Input: part model. Units: mm. Frame: model coordinates. Coordinates: 2 decimals unless noted, no trailing zeros. Order: outer loops, then holes, each group sorted by start corner. A loop starts at its lowest first (then second) coordinate and runs counter-clockwise, first axis right, second up. Notation, with made-up numbers: (-10, 28) -> (45, 28) arc R26 ccw to (45, 57) -> close; hole circle Ø5 at (52.25, 11). An arc over 180 degrees is marked (long way). Use one line per item in the form item = value. Start each with the question number.
1) Pin query (flat end, axial travel): pin 1 (3 mm diameter, centred on x = 4.5, y = -201, fed in from +Z); pin 2 (1.5 mm diameter, centred on x = 5, z = 2, fed in from -Y); pin 3 (1 mm diameter, centred on x = 5, z = 49, fed in from +Y). Return the tip coordinate at first contact, or that it passes through.
2) Section query A-A on x = 5.25. Output: boundary loops of the cut face in (y, z), then the cut area to 3 significant figures.
3) Section query B-B on y = -34. Output: boundary loops of the cut face in (x, z).
4) Section query C-C on z = 37. Output: boundary loops of the cut face in (x, y).
5) Ray query, line 1 along Z through (x, y) = (2.75, -2); line 2 along Z through (x, y) = (3.75, -242); line 3 along Y through (x, z) = (5.75, -4). Return the intervals inside material, ascending.
Autodesk Inventor part; units mm, degrees
ref_plane "YZ Plane" through (0, 0, 0) normal (1, 0, 0) x (0, 1, 0)
ref_plane "XZ Plane" through (0, 0, 0) normal (0, 1, 0) x (-1, 0, 0)
ref_plane "XY Plane" through (0, 0, 0) normal (0, 0, 1) x (1, 0, 0)
sketch "Sketch1" plane through (0, 0, 0) normal (1, 0, 0) x (0, 1, 0)
  circle A0 centre (0, 0) radius 3.175
  line L0 (0, 0) -> (12.7, 0)
  line L1 (0, 0) -> (12.7, 0) construction
  line L2 (12.7, 0) -> (12.7, -12.7)
  line L3 (12.7, -12.7) -> (-405.9936, -12.7)
  line L4 (-405.9936, -12.7) -> (-405.9936, 12.7)
  line L5 (-405.9936, 12.7) -> (12.7, 12.7)
  line L6 (12.7, 12.7) -> (12.7, -12.7)
  line L7 (-405.9936, 12.7) -> (-498.3106, 105.017)
  line L8 (-405.9936, 12.7) -> (-275.4376, 12.7) construction
  line L9 (-498.3106, 105.017) -> (-516.2711, 87.0565)
  line L10 (-516.2711, 87.0565) -> (-408.5081, -20.7066)
  line L11 (-405.9936, -12.7) -> (-431.3936, -12.7)
  line L12 (-405.9936, -12.7) -> (-380.5936, -12.7) construction
  line L13 (-516.2711, 87.0565) -> (-416.5146, -12.7)
  line L14 (-416.5146, -12.7) -> (12.7, -12.7)
  dimension "d0" = 6.35
  dimension "d1" = 12.7
  dimension "d2" = 0
  dimension "d3" = 12.7
  dimension "d4" = 90
  dimension "d5" = 418.6936
  dimension "d6" = 25.4
  dimension "d7" = 130.556
  dimension "d8" = 135
  dimension "d9" = 25.4
  dimension "d10" = 90
  dimension "d11" = 152.4
  dimension "d12" = 90
  dimension "d13" = 25.4
  dimension "d14" = 180
extrude "Extrusion1" add sketch "Sketch1" along normal blind 25.4
sketch "Sketch2" plane through (25.4, 0, 0) normal (1, 0, 0) x (0, 0, -1)
  line L0 (-105.017, -498.3106) -> (-87.0565, -516.2711)
  line L1 (-87.0565, -516.2711) -> (12.7, -416.5146)
  line L2 (-12.7, 12.7) -> (-12.7, -405.9936)
  line L3 (-96.0368, -507.2909) -> (-78.0763, -507.2909)
  line L4 (-105.017, -498.3106) -> (-100.5269, -502.8008)
  line L5 (-100.5269, -502.8008) -> (-73.5861, -502.8008)
  arc A0 (-100.5269, -502.8008) -> (-73.5861, -502.8008) centre (-87.0565, -489.3304) ccw
  dimension "d17" = 6.35
  dimension "d18" = 19.05
extrude "Extrusion2" cut sketch "Sketch2" against normal blind 25.4 contours A0 L3 L0 | L3 A0 L1 L0 | L1 L3 A0
sketch "Sketch3" plane through (0, 12.7, 12.7) normal (0, 1, 0) x (1, 0, 0)
  line L0 (0, 25.4) -> (0, 0)
  line L1 (0, 0) -> (25.4, 0)
  line L2 (25.4, 25.4) -> (25.4, 0)
  line L3 (0, 25.4) -> (25.4, 25.4)
  point P0 (0, 12.7)
extrude "Extrusion3" add sketch "Sketch3" along normal blind 127
sketch "Sketch4" plane through (25.4, 0, 0) normal (1, 0, 0) x (0, 0, -1)
  arc A0 (-100.5269, -502.8008) -> (-73.5861, -502.8008) centre (-87.0565, -489.3304) ccw
  line L0 (-73.5861, -502.8008) -> (12.7, -416.5146)
  line L1 (12.7, -416.5146) -> (12.7, 139.7)
  line L2 (-12.7, 139.7) -> (12.7, 139.7)
  line L3 (-12.7, -405.9936) -> (-12.7, 139.7)
  line L4 (-12.7, -405.9936) -> (-105.017, -498.3106)
  line L5 (-105.017, -498.3106) -> (-100.5269, -502.8008)
  circle A1 centre (0, 0) radius 3.175
extrude "Extrusion4" cut sketch "Sketch4" against normal blind 19.05
sketch "Sketch5" plane through (6.35, 0, 0) normal (1, 0, 0) x (0, 0, -1)
  line L0 (-12.7, 139.7) -> (12.7, 139.7)
  line L1 (12.7, 139.7) -> (12.7, 12.7)
  line L2 (12.7, 12.7) -> (-12.7, 12.7)
  line L3 (-12.7, 12.7) -> (-12.7, 139.7)
  dimension "d25" = 25.4
  dimension "d26" = 127
extrude "Extrusion5" cut sketch "Sketch5" against normal blind 127
sketch "Sketch8" plane through (6.35, 12.7, 12.7) normal (0, 1, 0) x (1, 0, 0)
  line L0 (-6.35, 0) -> (-6.35, 25.4)
  line L1 (0, 0) -> (-6.35, 0)
  line L2 (0, 25.4) -> (0, 0)
  line L3 (-6.35, 25.4) -> (0, 25.4)
  point P0 (-6.35, 12.7)
extrude "Extrusion8" add sketch "Sketch8" along normal blind 101.6
sketch "Sketch9" plane through (6.35, 0, 0) normal (1, 0, 0) x (0, 0, -1)
  circle A0 centre (0, 0) radius 3.175
  circle A1 centre (0, 0) radius 6.35
  dimension "d45" = 12.7
extrude "Extrusion9" cut sketch "Sketch9" against normal blind 25.4
sketch "Sketch10" plane through (6.35, 0, 0) normal (1, 0, 0) x (0, 0, -1)
  circle A0 centre (0, 0) radius 6.35
  line L0 (-5.5563, -5.5563) -> (5.5563, -5.5563)
  line L1 (5.5563, -5.5563) -> (5.5563, 5.5563)
  line L2 (5.5563, 5.5563) -> (-5.5563, 5.5563)
  line L3 (-5.5563, 5.5563) -> (-5.5563, -5.5563)
  line L4 (-5.5563, -5.5563) -> (5.5563, 5.5563) construction
  line L5 (5.5563, -5.5563) -> (-5.5563, 5.5563) construction
  line L6 (5.5563, -3.0742) -> (0.1158, -6.3489)
  line L7 (0.1158, -6.3489) -> (-5.4404, -3.2748)
  line L8 (-5.4404, -3.2748) -> (-5.5563, 3.0742)
  line L9 (-5.5563, 3.0742) -> (-0.1158, 6.3489)
  line L10 (-0.1158, 6.3489) -> (5.4404, 3.2748)
  line L11 (5.4404, 3.2748) -> (5.5563, -3.0742)
  dimension "d48" = 11.1125
  dimension "d49" = 11.1125
extrude "Extrusion10" add sketch "Sketch10" against normal blind 6.35 contours L1 A0 | L11 A0 L1 | A0 L0 L6 | A0 L6 L0 | L10 L2 A0 | A0 L0 L7 | L0 A0 L7 | L2 L10 A0 | A0 L3 L8 | L9 L2 A0 | L9 A0 L2 | A0 L3
properties part number "FlatArm"
Answers below:
q1.pin_1 = 12.7
q1.pin_2 = -431.96
q1.pin_3 = -441.79
q2.outline = (-502.8, 73.59) -> (-416.51, -12.7) -> (114.3, -12.7) -> (114.3, 12.7) -> (-405.99, 12.7) -> (-498.31, 105.02) -> (-502.8, 100.53) arc R19.05 ccw to start; hole (-6.35, -0.12) -> (-3.07, -5.56) -> (3.27, -5.44) -> (6.35, 0.12) -> (3.07, 5.56) -> (-3.27, 5.44) -> close
q2.area = 16,600 mm^2
q3.outline = (0, -12.7) -> (6.35, -12.7) -> (6.35, 12.7) -> (0, 12.7) -> close
q4.outline = (0, -466.21) -> (6.35, -466.21) -> (6.35, -430.29) -> (0, -430.29) -> close
q5.line_1 = -12.7 to -5.54, 5.46 to 12.7
q5.line_2 = -12.7 to 12.7
q5.line_3 = -425.21 to -4.01, 4.07 to 114.3
